Can you work these out from the model? Positions are in its coordinate system, mm. Coordinates: 2 decimals unless noted, no trailing zeros. Order: outer loops, then holes, each group sorted by start corner. A loop starts at its lowest first (then second) coordinate and runs counter-clockwise, first axis right, second up. Notation, with made-up numbers: (55, 21) -> (80, 21) arc R20 ccw to (80, 34) -> close; hole circle Ø8 at (-34, -38). An arc over 180 degrees is marked (long way). Answer as a JSON object with one key per item and string values. Group by question number.
(1) For pin 1 (4 mm diameter, centred on x = -7.5, z = 51, fed in from +Y); pin 2 (1 mm diameter, centred on x = -7.5, y = 5.5, fed in from +Z); pin 3 (1 mm diameter, centred on x = -4, z = 191.5, fed in from -Y), each with a flat end and sliding along its axis, tell me the tip position at first contact or that it passes through.
(2) I want a section at A-A, the plane z = 335.5. List the corners of the cut face in (x, y) for me, plus the area to 3 significant figures.
(3) I need wall thicknesses on line 1 (Y direction, x = 1, z = 350.5); line 2 (X direction, y = -1, z = 261.5); line 3 (X direction, y = 0.5, z = 307). Which ranges of each line are inside material? Lowest first, please.
Solid Edge part; units mm, degrees
sketch "Sketch1" plane through (0, 0, 0) normal (0, 0, 1) x (1, 0, 0)
  line L0 (12.5, 2.5) -> (9.6825, 2.5)
  line L1 (12.5, -2.5) -> (12.5, 2.5)
  line L2 (9.6825, -2.5) -> (12.5, -2.5)
  arc A0 (9.6825, -2.5) -> (9.6825, 2.5) centre (0, 0) cw
extrude "Protrusion1" add sketch "Sketch1" along normal blind 457.2
sketch "Sketch2" plane through (0, 0, 0) normal (0, 0, 1) x (1, 0, 0)
  line L0 (12.5, 2.5) -> (9.6825, 2.5)
  line L1 (12.5, -2.5) -> (12.5, 2.5)
  line L2 (9.6825, -2.5) -> (12.5, -2.5)
  arc A0 (9.6825, -2.5) -> (9.6825, 2.5) centre (0, 0) cw
sketch "Sketch3" plane through (0, 0, 0) normal (0, -1, 0) x (1, 0, 0)
  line L0 (11.0912, 0) -> (12.5, 1.4088)
  line L1 (12.5, 1.4088) -> (12.5, 0)
  line L2 (12.5, 0) -> (11.0912, 0)
sweep "SweptCutout_1" cut profiles "Sketch3" path "Sketch2"
sketch "Sketch4" plane through (0, 0, 0) normal (0, -1, 0) x (1, 0, 0)
  line L0 (12.5, 457.2) -> (12.5, 455.7912)
  line L1 (11.0912, 457.2) -> (12.5, 455.7912)
  line L2 (11.0912, 457.2) -> (12.5, 457.2)
sketch3d "SweptCutout_2 path"
  arc A0 (9.6825, -2.5, 457.2) -> (-10, 0, 457.2) centre (0, 0, 457.2)
  arc A1 (-10, 0, 457.2) -> (9.6825, 2.5, 457.2) centre (0, 0, 457.2)
  line L2 (9.6825, -2.5, 457.2) -> (12.5, -2.5, 457.2)
  line L3 (12.5, -2.5, 457.2) -> (12.5, 2.5, 457.2)
  line L4 (12.5, 2.5, 457.2) -> (9.6825, 2.5, 457.2)
sweep "SweptCutout_2" cut profiles "Sketch4" path "SweptCutout_2 path"
Computed values:
{
 "1": {"pin 1": "stops at y = 8.35", "pin 2": "stops at z = 456.99", "pin 3": "stops at y = -9.37"},
 "2": {"outline": "(9.68, -2.5) -> (12.5, -2.5) -> (12.5, 2.5) -> (9.68, 2.5) arc R10 ccw (long way) to start", "area": "327 mm2"},
 "3": {"line 1": "y = -9.95 to 9.95", "line 2": "x = -9.95 to 12.5", "line 3": "x = -9.99 to 12.5"}
}
